The listing builds one solid part. Answer for the finished solid, in the listing's coordinates (mm). A direction names the side the tool comes from. Coordinates: 2 decimals unless noted, no trailing zeros. Loops run counter-clockwise (first coordinate to the right, second up) from the corner with the lowest first, then second, coordinate; pieces in that order, holes last. Notation, with made-up numbers: (40, 76) - (53, 76) arc R24 ccw to (53, 114) - close; hole circle Ø7 at (46.5, 23). An arc over 180 degrees is marked (long way). Return JSON: item names as keys, results as strings. Group by question number.
1. Section D-D (x = -5.75) is taken. Write down the section's boundary in (y, z), and give its area (3 significant figures).
2. Section A-A (x = 0) is taken. Write down the section's boundary in (y, z).
3. The mould has two halves that part along Z. Classify faces 4 (the face through (0, -23.5, -0.75)), 5 (the face through (-10.5, -3, -2)), 6 (the face through (0, -23.5, -4.75)), 7 (the face through (0, -8, 2)): pulls with the +Z half, pulls with the -Z half, needs draft (parallel to the pull), parting line crosses it, or undercut.
4. Section B-B (y = -15) is taken. Write down the section's boundary in (x, z), and give its area (3 significant figures).
5. Find the intervals of material crossed by line 1 along X through (y, z) = (-24.25, -2.75); line 2 along X through (y, z) = (-5, -3.75); line 3 along X through (y, z) = (15, 0.2), in increasing order.
6. Each of these flat-tipped pins is pushed along its axis until it touches: P1, Ø2.5, axis at x = -8, y = 15, coming from the -Z side; P2, Ø1.2, axis at x = 11.5, y = 6.5, coming from the -Z side; P3, Ø3.5, axis at x = 8, y = 15.5, coming from the +Z side; P4, Ø1.8, axis at x = -8, y = -15, coming from the +Z side. Where does it stop, or does it pass through?
7. Which of the six approach directions +Z, -Z, +X, -X, +Y, -Y give full straight-line access (tool end or side, diameter ignored) to faces 1 (the face through (-8, 14, 1)), 2 (the face through (-1.724, -23.493, -3.764)), 3 (the face through (-5, -24, -3))?
8. Section C-C (y = 15) is taken. Write down the section's boundary in (x, z).
```python
from build123d import *

# Parameters (mm, degrees)
SKETCH1_W                  = 21
SKETCH1_H                  = 35
SKETCH1_R                  = 0.8
SKETCH1_R_2                = 8.5
BRACKETWITHBOLTHOLES_DEPTH = 2
SKETCH2_W                  = 10
SKETCH2_H                  = 2
BRACKETEXTENSION_DEPTH     = 2
SKETCH2_3_W                = 10
SKETCH2_3_H                = 2
BASE_DEPTH                 = 7.5
SKETCH3_R                  = 1
BASEBOLTHOLE_DEPTH         = 3
BASENUTSLOT_DEPTH          = 1
STIFFENERRIB_DEPTH         = 42.5
SKETCH5_R                  = 1.5
BOLTHATSLOTS_DEPTH         = 1


with BuildPart() as part:
    # Sketch1 → BracketWithBoltHoles (new body)
    with BuildSketch(Plane.XY):
        Rectangle(SKETCH1_W, SKETCH1_H)
        with Locations((-8, 15)):
            Circle(SKETCH1_R, mode=Mode.SUBTRACT)
        with Locations((8, 15)):
            Circle(SKETCH1_R, mode=Mode.SUBTRACT)
        with Locations((8, -15)):
            Circle(SKETCH1_R, mode=Mode.SUBTRACT)
        with Locations((-8, -15)):
            Circle(SKETCH1_R, mode=Mode.SUBTRACT)
        with Locations((0, 7.5)):
            Circle(SKETCH1_R_2, mode=Mode.SUBTRACT)
    extrude(amount=BRACKETWITHBOLTHOLES_DEPTH)

    # Sketch2 → BracketExtension (add)
    with BuildSketch(Plane.XY.offset(2)):
        Polygon((10.5, -17.5), (-10.5, -17.5), (-10.5, -25), (-5, -25), (-5, -23), (5, -23), (5, -25), (10.5, -25), align=None)
        with Locations((0, -24)):
            Rectangle(SKETCH2_W, SKETCH2_H)
    extrude(amount=-BRACKETEXTENSION_DEPTH)

    # Sketch2<3> → Base (add)
    with BuildSketch(Plane.XY.offset(2)):
        with Locations((0, -24)):
            Rectangle(SKETCH2_3_W, SKETCH2_3_H)
    extrude(amount=-BASE_DEPTH)

    # Sketch3 → BaseBoltHole (cut, through all)
    with BuildSketch(Plane(origin=(0, -23, 0), x_dir=(1, 0, 0), z_dir=(0, 1, 0))):
        with Locations((0, 2.75)):
            Circle(SKETCH3_R)
    extrude(amount=-BASEBOLTHOLE_DEPTH, mode=Mode.SUBTRACT)

    # Sketch3<3> → BaseNutSlot (cut)
    with BuildSketch(Plane(origin=(0, -23, 0), x_dir=(1, 0, 0), z_dir=(0, 1, 0))):
        Polygon((2.309401077, 2.75), (1.154700538, 4.75), (-1.154700538, 4.75), (-2.309401077, 2.75), (-1.154700538, 0.75), (1.154700538, 0.75), align=None)
    extrude(amount=-BASENUTSLOT_DEPTH, mode=Mode.SUBTRACT)

    # Sketch4 → StiffenerRib (add)
    with BuildSketch(Plane(origin=(0, 17.5, 0), x_dir=(1, 0, 0), z_dir=(0, 1, 0))):
        Polygon((-10.5, 4), (-12, 4), (-12, -2), (-10.5, -2), (-10.5, 0), align=None)
    stiffenerrib = extrude(amount=-STIFFENERRIB_DEPTH)

    # StiffenerRib2: StiffenerRib across plane
    add(stiffenerrib.mirror(Plane(origin=(0, 0, 0), x_dir=(0, 0, 1), z_dir=(1, 0, 0))))

    # Sketch5 → BoltHatSlots (cut)
    with BuildSketch(Plane.XY.offset(2)):
        with Locations((8, 15)):
            Circle(SKETCH5_R)
        with Locations((8, -15)):
            Circle(SKETCH5_R)
        with Locations((-8, -15)):
            Circle(SKETCH5_R)
        with Locations((-8, 15)):
            Circle(SKETCH5_R)
    extrude(amount=-BOLTHATSLOTS_DEPTH, mode=Mode.SUBTRACT)


solid = part.part
```
The answers:
{
 "1": {"outline": "(-25, 0) - (1.24, 0) - (1.24, 2) - (-25, 2) - close; (13.76, 0) - (17.5, 0) - (17.5, 2) - (13.76, 2) - close", "area": "60.0 mm2"},
 "2": {"outline": "(-25, -5.5) - (-23, -5.5) - (-23, -4.75) - (-24, -4.75) - (-24, -3.75) - (-25, -3.75) - close; (-25, -1.75) - (-24, -1.75) - (-24, -0.75) - (-23, -0.75) - (-23, 0) - (-1, 0) - (-1, 2) - (-25, 2) - close; (16, 0) - (17.5, 0) - (17.5, 2) - (16, 2) - close"},
 "3": {"face 4": "undercut", "face 5": "needs draft", "face 6": "undercut", "face 7": "pulls with the +Z half"},
 "4": {"outline": "(-12, -4) - (-10.5, -4) - (-10.5, 0) - (-8.8, 0) - (-8.8, 1) - (-9.5, 1) - (-9.5, 2) - (-12, 2) - close; (-7.2, 0) - (7.2, 0) - (7.2, 1) - (6.5, 1) - (6.5, 2) - (-6.5, 2) - (-6.5, 1) - (-7.2, 1) - close; (8.8, 0) - (10.5, 0) - (10.5, -4) - (12, -4) - (12, 2) - (9.5, 2) - (9.5, 1) - (8.8, 1) - close", "area": "50.8 mm2"},
 "5": {"line 1": "x = -12 to -10.5, -5 to -1, 1 to 5, 10.5 to 12", "line 2": "x = -12 to -10.5, 10.5 to 12", "line 3": "x = -12 to -8.8, -7.2 to -4, 4 to 7.2, 8.8 to 12"},
 "6": {"P1": "stops at z = 0", "P2": "stops at z = -4", "P3": "stops at z = 2", "P4": "stops at z = 1"},
 "7": {"face 1": "+Z", "face 2": "+Y", "face 3": "-Z, +Y, -Y"},
 "8": {"outline": "(-12, -4) - (-10.5, -4) - (-10.5, 0) - (-8.8, 0) - (-8.8, 1) - (-9.5, 1) - (-9.5, 2) - (-12, 2) - close; (-7.2, 0) - (-4, 0) - (-4, 2) - (-6.5, 2) - (-6.5, 1) - (-7.2, 1) - close; (4, 0) - (7.2, 0) - (7.2, 1) - (6.5, 1) - (6.5, 2) - (4, 2) - close; (8.8, 0) - (10.5, 0) - (10.5, -4) - (12, -4) - (12, 2) - (9.5, 2) - (9.5, 1) - (8.8, 1) - close"}
}
